Source: CAD feature listing. Evaluate the final solid. Frame: model axes, mm. A direction names the side the tool comes from. Give positions to 0.01 mm unless a question says otherwise; leave off trailing zeros. Write each loop counter-clockwise with the first axis right and the second up, starting at its lowest first coordinate (ties: lowest second). Pieces come first, ordered by that corner, then holes. Notation, with made-up numbers: M -36.75,49.5 L -12.75,49.5 A28 cw -12.75,83.5 Z; hole C 72,2 d11. An arc over 180 degrees is marked long. Answer as a JSON object with one key per item and string values. Group by question number.
```python
from build123d import *

# Parameters (mm, degrees)
SKETCH1_R            = 7.5
SKETCH1_R_2          = 2.5
BOSS_EXTRUDE1_DEPTH  = 5.4
BOSS_EXTRUDE2_START  = 5.4
SKETCH2_R            = 7.5
SKETCH2_R_2          = 2.5
BOSS_EXTRUDE2_DEPTH  = 5.4
BOSS_EXTRUDE3_START  = 5.4
SKETCH3_R            = 7.5
SKETCH3_R_2          = 2.5
BOSS_EXTRUDE3_DEPTH  = 5.4
BOSS_EXTRUDE4_START  = 5.4
SKETCH4_R            = 7.5
SKETCH4_R_2          = 2.5
BOSS_EXTRUDE4_DEPTH  = 5.4
BOSS_EXTRUDE5_START  = 5.4
SKETCH5_R            = 7.5
SKETCH5_R_2          = 2.5
BOSS_EXTRUDE5_DEPTH  = 5.4
BOSS_EXTRUDE6_START  = 5.4
SKETCH6_R            = 7.5
SKETCH6_R_2          = 2.5
BOSS_EXTRUDE6_DEPTH  = 5.4
BOSS_EXTRUDE7_START  = 5.4
SKETCH7_R            = 7.5
SKETCH7_R_2          = 2.5
BOSS_EXTRUDE7_DEPTH  = 5.4
BOSS_EXTRUDE9_START  = 5.4
SKETCH8_R            = 7.5
SKETCH8_R_2          = 2.5
BOSS_EXTRUDE9_DEPTH  = 5.4
BOSS_EXTRUDE10_START = 5.4
SKETCH9_R            = 7.5
SKETCH9_R_2          = 2.5
BOSS_EXTRUDE10_DEPTH = 5.4
BOSS_EXTRUDE11_START = 5.4
SKETCH10_R           = 7.5
SKETCH10_R_2         = 2.5
BOSS_EXTRUDE11_DEPTH = 5.4
BOSS_EXTRUDE12_START = 5.4
SKETCH11_R           = 7.5
SKETCH11_R_2         = 2.5
BOSS_EXTRUDE12_DEPTH = 5.4
BOSS_EXTRUDE13_START = 5.4
SKETCH12_R           = 7.5
SKETCH12_R_2         = 2.5
BOSS_EXTRUDE13_DEPTH = 5.4
BOSS_EXTRUDE14_START = 5.4
SKETCH13_R           = 7.5
SKETCH13_R_2         = 2.5
BOSS_EXTRUDE14_DEPTH = 5.4
SKETCH14_R           = 2.5
BOSS_EXTRUDE15_DEPTH = 80
BOSS_EXTRUDE16_START = 30
SKETCH14_2_R         = 2.5
BOSS_EXTRUDE16_DEPTH = 30
SKETCH15_R           = 7
BOSS_EXTRUDE17_DEPTH = 13


with BuildPart() as part:
    # Sketch1 → Boss-Extrude1 (new body)
    with BuildSketch(Plane.XY):
        with Locations(Location((0, 2, 0), (0, 0, 180))):
            Circle(SKETCH1_R)
        with Locations(Location((0, 0, 0), (0, 0, 180))):
            Circle(SKETCH1_R_2, mode=Mode.SUBTRACT)
    extrude(amount=BOSS_EXTRUDE1_DEPTH)

    # Sketch2 → Boss-Extrude2 (add)
    with BuildSketch(Plane(origin=(0, 0, 0), x_dir=(-1, 0, 0), z_dir=(0, 0, -1)).offset(BOSS_EXTRUDE2_START)):
        with Locations(Location((-1, 1.732050808, 0), (0, 0, 101.042389991))):
            Circle(SKETCH2_R)
        Circle(SKETCH2_R_2, mode=Mode.SUBTRACT)
    extrude(amount=-BOSS_EXTRUDE2_DEPTH)

    # Sketch3 → Boss-Extrude3 (add)
    with BuildSketch(Plane(origin=(0, 0, -5.4), x_dir=(-1, 0, 0), z_dir=(0, 0, -1)).offset(BOSS_EXTRUDE3_START)):
        with Locations(Location((-1.732050808, 1, 0), (0, 0, 131.042389991))):
            Circle(SKETCH3_R)
        Circle(SKETCH3_R_2, mode=Mode.SUBTRACT)
    extrude(amount=-BOSS_EXTRUDE3_DEPTH)

    # Sketch4 → Boss-Extrude4 (add)
    with BuildSketch(Plane(origin=(0, 0, -10.8), x_dir=(-1, 0, 0), z_dir=(0, 0, -1)).offset(BOSS_EXTRUDE4_START)):
        with Locations(Location((-2, 0, 0), (0, 0, 161.042389991))):
            Circle(SKETCH4_R)
        Circle(SKETCH4_R_2, mode=Mode.SUBTRACT)
    extrude(amount=-BOSS_EXTRUDE4_DEPTH)

    # Sketch5 → Boss-Extrude5 (add)
    with BuildSketch(Plane(origin=(0, 0, -16.2), x_dir=(-1, 0, 0), z_dir=(0, 0, -1)).offset(BOSS_EXTRUDE5_START)):
        with Locations(Location((-1.732050808, -1, 0), (0, 0, 191.042389991))):
            Circle(SKETCH5_R)
        Circle(SKETCH5_R_2, mode=Mode.SUBTRACT)
    extrude(amount=-BOSS_EXTRUDE5_DEPTH)

    # Sketch6 → Boss-Extrude6 (add)
    with BuildSketch(Plane(origin=(0, 0, -21.6), x_dir=(-1, 0, 0), z_dir=(0, 0, -1)).offset(BOSS_EXTRUDE6_START)):
        with Locations(Location((-1, -1.732050808, 0), (0, 0, 221.042389991))):
            Circle(SKETCH6_R)
        Circle(SKETCH6_R_2, mode=Mode.SUBTRACT)
    extrude(amount=-BOSS_EXTRUDE6_DEPTH)

    # Sketch7 → Boss-Extrude7 (add)
    with BuildSketch(Plane(origin=(0, 0, -27), x_dir=(-1, 0, 0), z_dir=(0, 0, -1)).offset(BOSS_EXTRUDE7_START)):
        with Locations(Location((0, -2, 0), (0, 0, 251.042389991))):
            Circle(SKETCH7_R)
        Circle(SKETCH7_R_2, mode=Mode.SUBTRACT)
    extrude(amount=-BOSS_EXTRUDE7_DEPTH)

    # Sketch8 → Boss-Extrude9 (add)
    with BuildSketch(Plane(origin=(0, 0, -32.4), x_dir=(-1, 0, 0), z_dir=(0, 0, -1)).offset(BOSS_EXTRUDE9_START)):
        with Locations(Location((1, -1.732050808, 0), (0, 0, 108.957610009))):
            Circle(SKETCH8_R)
        Circle(SKETCH8_R_2, mode=Mode.SUBTRACT)
    extrude(amount=-BOSS_EXTRUDE9_DEPTH)

    # Sketch9 → Boss-Extrude10 (add)
    with BuildSketch(Plane(origin=(0, 0, -37.8), x_dir=(-1, 0, 0), z_dir=(0, 0, -1)).offset(BOSS_EXTRUDE10_START)):
        with Locations(Location((1.732050808, -1, 0), (0, 0, 138.957610009))):
            Circle(SKETCH9_R)
        Circle(SKETCH9_R_2, mode=Mode.SUBTRACT)
    extrude(amount=-BOSS_EXTRUDE10_DEPTH)

    # Sketch10 → Boss-Extrude11 (add)
    with BuildSketch(Plane(origin=(0, 0, -43.2), x_dir=(-1, 0, 0), z_dir=(0, 0, -1)).offset(BOSS_EXTRUDE11_START)):
        with Locations(Location((2, 0, 0), (0, 0, 168.957610009))):
            Circle(SKETCH10_R)
        Circle(SKETCH10_R_2, mode=Mode.SUBTRACT)
    extrude(amount=-BOSS_EXTRUDE11_DEPTH)

    # Sketch11 → Boss-Extrude12 (add)
    with BuildSketch(Plane(origin=(0, 0, -48.6), x_dir=(-1, 0, 0), z_dir=(0, 0, -1)).offset(BOSS_EXTRUDE12_START)):
        with Locations(Location((1.732050808, 1, 0), (0, 0, 198.957610009))):
            Circle(SKETCH11_R)
        Circle(SKETCH11_R_2, mode=Mode.SUBTRACT)
    extrude(amount=-BOSS_EXTRUDE12_DEPTH)

    # Sketch12 → Boss-Extrude13 (add)
    with BuildSketch(Plane(origin=(0, 0, -54), x_dir=(-1, 0, 0), z_dir=(0, 0, -1)).offset(BOSS_EXTRUDE13_START)):
        with Locations(Location((1, 1.732050808, 0), (0, 0, 228.957610009))):
            Circle(SKETCH12_R)
        Circle(SKETCH12_R_2, mode=Mode.SUBTRACT)
    extrude(amount=-BOSS_EXTRUDE13_DEPTH)

    # Sketch13 → Boss-Extrude14 (add)
    with BuildSketch(Plane(origin=(0, 0, -59.4), x_dir=(-1, 0, 0), z_dir=(0, 0, -1)).offset(BOSS_EXTRUDE14_START)):
        with Locations(Location((0, 2, 0), (0, 0, 281.042389991))):
            Circle(SKETCH13_R)
        Circle(SKETCH13_R_2, mode=Mode.SUBTRACT)
    extrude(amount=-BOSS_EXTRUDE14_DEPTH)

    # Sketch14 → Boss-Extrude15 (add)
    with BuildSketch(Plane(origin=(0, 0, -64.8), x_dir=(-1, 0, 0), z_dir=(0, 0, -1))):
        Circle(SKETCH14_R)
    extrude(amount=-BOSS_EXTRUDE15_DEPTH)

    # Sketch14_2 → Boss-Extrude16 (add)
    with BuildSketch(Plane(origin=(0, 0, -64.8), x_dir=(-1, 0, 0), z_dir=(0, 0, -1)).offset(BOSS_EXTRUDE16_START)):
        Circle(SKETCH14_2_R)
    extrude(amount=-BOSS_EXTRUDE16_DEPTH)

    # Sketch15 → Boss-Extrude17 (add)
    with BuildSketch(Plane(origin=(0, 0, -64.8), x_dir=(-1, 0, 0), z_dir=(0, 0, -1))):
        with Locations(Location((0, 0, 0), (0, 0, 186.665427256))):
            Circle(SKETCH15_R)
    extrude(amount=BOSS_EXTRUDE17_DEPTH)


solid = part.part
```
(1) Ray query, L1, parallel to Z at x = -7, y = 2.5; L2, parallel to Z at x = 0.75, y = 7.5; L3, parallel to Z at x = 4, y = 3.5. Return the intervals inside material, ascending. Write a range as [from, to].
(2) Section B-B, the plane z = -76. Return loops of the section in (x, y), plus the area to 3 significant figures.
(3) Section A-A, the plane z = -7.5. Return loops of the section in (x, y).
(4) Contact query for flat-ended pins moving along their axis: pin 1 Ø5 at (x, z) = (-5, -65) entering from +Y; pin 2 Ø1 at (x, y) = (0.5, -3) entering from +Z; pin 3 Ø6 at (x, z) = (-7.5, 3) entering from -Y. Output: stop coordinate, or through.
(5) Pull-direction query (Z, two-part tool) for faces 1 (the flat face through (0, 0, -94.8)), 2 (the flat face through (6.2, 4.4, -59.4)), 3 (the cylindrical face through (0.54, -2.44, 10.23)), 4 (the flat face through (7.2, 0.7, -27)); classes: pulls with the +Z half, pulls with the -Z half, needs draft (parallel to the pull), parting line crosses it, or undercut.
(6) Access query for faces 5 (the cylindrical face through (-0.65, -8.11, -18.94)), 6 (the cylindrical face through (-4.032, -4.324, 2.662)). Directions: +Z, -Z, +X, -X, +Y, -Y. A direction counts if a zero-diameter tool reaches every point of the face in a straight line with its end or side. Return the directions, or none.
Reported:
{
 "1": {"L1": "z = [-64.8, -32.4], [0, 5.4]", "L2": "z = [-64.8, -48.6], [-10.8, 5.4]", "L3": "z = [-77.8, 5.4]"},
 "2": {"outline": "C 0,0 d14", "area": "154 mm2"},
 "3": {"outline": "C 1.73,1 d15"},
 "4": {"pin 1": "stops at y = 9.07", "pin 2": "stops at z = 5.4", "pin 3": "stops at y = -4"},
 "5": {"face 1": "pulls with the -Z half", "face 2": "undercut", "face 3": "needs draft", "face 4": "undercut"},
 "6": {"face 5": "none", "face 6": "+Z"}
}
